Read the model definition and answer for the solid it produces. Units are mm, in the model's axes. A direction names the side the tool comes from. Round coordinates to 2 decimals unless told otherwise and drop trailing zeros. Order: outer loops, then holes, each group sorted by start corner. A loop starts at its lowest first (then second) coordinate and runs counter-clockwise, first axis right, second up.
from build123d import *

# Parameters (mm, degrees)
CROQUIS1_W              = 110
CROQUIS1_H              = 220
SALIENTE_EXTRUIR1_DEPTH = 6.35
CROQUIS2_R              = 2
CORTAR_EXTRUIR2_DEPTH   = 7.35


with BuildPart() as part:
    # Croquis1 → Saliente-Extruir1 (new body)
    with BuildSketch(Plane.XY):
        Rectangle(CROQUIS1_W, CROQUIS1_H)
    extrude(amount=SALIENTE_EXTRUIR1_DEPTH)

    # Croquis2 → Cortar-Extruir2 (cut, through all)
    with BuildSketch(Plane.XY):
        with Locations((40, 106.825)):
            Circle(CROQUIS2_R)
        with Locations((-40, 106.825)):
            Circle(CROQUIS2_R)
        with Locations((0, 106.825)):
            Circle(CROQUIS2_R)
        with BuildLine():
            Line((15, -52), (15, -102))
            ThreePointArc((15, -102), (19.408343114, -106.964870807), (24.859976852, -103.175))
            Line((24.859976852, -103.175), (25, -52))
            ThreePointArc((25, -52), (20, -47), (15, -52))
        make_face()
        with BuildLine():
            Line((-25, -52), (-25, -102))
            ThreePointArc((-25, -102), (-20, -107), (-15, -102))
            Line((-15, -102), (-15, -52))
            ThreePointArc((-15, -52), (-20, -47), (-25, -52))
        make_face()
    extrude(amount=CORTAR_EXTRUIR2_DEPTH, mode=Mode.SUBTRACT)


solid = part.part
Q1. A cutting plane is placed at A-A, the plane x = 0. Give the vertices of the cut face in (y, z) (3 decimals), plus the area to 3 significant figures.
Outcome:
outline: (-110, 0) - (104.825, 0) - (104.825, 6.35) - (-110, 6.35) - close; (108.825, 0) - (110, 0) - (110, 6.35) - (108.825, 6.35) - close
area: 1,370 mm2
Q2. Straight lines are drawn through the part: probe 1 along X at (y, z) = (-67, 4.5); probe 2 along X at (y, z) = (-91, 6.25); probe 3 along Y at (x, z) = (-40, 5) (3 decimals). For each, find the intervals that lie inside material, in ascending order.
Outcome:
probe 1: x = -55 to -25, -15 to 15, 24.96 to 55
probe 2: x = -55 to -25, -15 to 15, 24.89 to 55
probe 3: y = -110 to 104.825, 108.825 to 110
Q3. A flat-ended cylindrical pin translates along its axis: pin 1 (3.5 mm diameter, centred on x = -40, y = 106.825, fed in from -Z). Find the tip coordinate at first contact, or state that the pin passes through.
Outcome:
pin 1: passes through
Q4. For faces 1 (the face through (55, -2, 3)), 2 (the face through (-25, -77, 3)), determine the directions among +Z, -Z, +X, -X, +Y, -Y from which every point of the face is accessible in a straight line to the end or side of a thin tool.
Outcome:
face 1: +Z, -Z, +X, +Y, -Y
face 2: +Z, -Z
Q5. For a pull along Y with two mould halves and no side action, classify faces 3 (the face through (-1, -110, 3)), 4 (the face through (-1, 110, 3)), 5 (the face through (20, -47, 3)), 6 (the face through (-1, 2, 0)) as released by +Y, released by -Y, zero draft, split by the parting line, or undercut.
Outcome:
face 3: released by -Y
face 4: released by +Y
face 5: undercut
face 6: zero draft
Q6. A cutting plane is placed at B-B, the plane y = -66.5. Give the vertices of the cut face in (x, z).
Outcome:
outline: (-55, 0) - (-25, 0) - (-25, 6.35) - (-55, 6.35) - close; (-15, 0) - (15, 0) - (15, 6.35) - (-15, 6.35) - close; (24.96, 0) - (55, 0) - (55, 6.35) - (24.96, 6.35) - close
Q7. A cutting plane is placed at C-C, the plane z = 4.25. Give the vertices of the cut face in (x, y) (3 decimals).
Outcome:
outline: (-55, -110) - (55, -110) - (55, 110) - (-55, 110) - close; hole circle Ø4 at (-40, 106.825); hole (-25, -102) arc R5 ccw to (-15, -102) - (-15, -52) arc R5 ccw to (-25, -52) - close; hole circle Ø4 at (0, 106.825); hole (15, -102) arc R5 ccw to (24.86, -103.175) - (25, -52) arc R5 ccw to (15, -52) - close; hole circle Ø4 at (40, 106.825)
